from build123d import *

# Parameters (mm, degrees)
SKETCH_1_R             = 19.1
EXTRUDE_1_DEPTH        = 40
SKETCH_2_R             = 5
EXTRUDE_2_DEPTH        = 17
CUT_EXTRUDE_START      = -15
CUT_EXTRUDE_1_DEPTH    = 15
HOLE_WIZARD_M3_1_D     = 2.5
HOLE_WIZARD_M3_1_DEPTH = 8.5
HOLE_WIZARD_M3_1_TIP   = 0.721687836


with BuildPart() as part:
    # 草图1 → 凸台-拉伸1 (new body)
    with BuildSketch(Plane(origin=(0, 0, 0), x_dir=(1, 0, 0), z_dir=(0, 1, 0))):
        with Locations(Location((0, 0, 0), (0, 0, 270))):
            Circle(SKETCH_1_R)
    extrude(amount=EXTRUDE_1_DEPTH)

    # 草图2 → 凸台-拉伸2 (add)
    with BuildSketch(Plane(origin=(0, 40, 0), x_dir=(1, 0, 0), z_dir=(0, 1, 0))):
        with Locations(Location((0, 0, 0), (0, 0, 270))):
            Circle(SKETCH_2_R)
    extrude(amount=EXTRUDE_2_DEPTH)

    # 草图3 → 切除-拉伸1 (cut)
    with BuildSketch(Plane(origin=(0, 57, 0), x_dir=(1, 0, 0), z_dir=(0, 1, 0)).offset(CUT_EXTRUDE_START)):
        with BuildLine():
            Line((-3, 4), (3, 4))
            ThreePointArc((3, 4), (0, 5), (-3, 4))
        make_face()
    extrude(amount=CUT_EXTRUDE_1_DEPTH, mode=Mode.SUBTRACT)

    # M3 螺纹孔1
    with Locations(Plane(origin=(0, 40, -15), x_dir=(0, 0, 1), z_dir=(0, 1, 0))):
        with Locations((0, 0), (15, -15), (15, 15), (30, 0)):
            Hole(HOLE_WIZARD_M3_1_D / 2, depth=HOLE_WIZARD_M3_1_DEPTH)
            with Locations((0, 0, -(HOLE_WIZARD_M3_1_DEPTH + HOLE_WIZARD_M3_1_TIP / 2))):  # 120° drill point
                Cone(0, HOLE_WIZARD_M3_1_D / 2, HOLE_WIZARD_M3_1_TIP, mode=Mode.SUBTRACT)


solid = part.part
Design review of the part built by this model. Coordinates are the model's own, in mm. A direction names the side the tool comes from. Give positions to 0.01 mm unless a question says otherwise; leave off trailing zeros. Loops run counter-clockwise (first coordinate to the right, second up) from the corner with the lowest first, then second, coordinate; pieces in that order, holes last. Notation, with made-up numbers: M -15.75,84.5 L -2.75,84.5 A14 ccw -2.75,93.5 Z; hole C 31.25,66.5 d8. An arc over 180 degrees is marked long. One line per question, with ' | ' between items. Start each with the question number.
1. Add section D-D (y = 4.5). Write out the cut boundary in (x, z), plus the area to 3 significant figures.
2. For faces 4 (the face through (0, 0, 0)), 5 (the face through (0.05, 35.69, -13.75)), list the 3-axis set-ups (+Z, -Z, +X, -X, +Y, -Y) from which the entire face can be reached by the end or side of a thin tool; tool diameter is ignored.
3. Add section C-C (z = 9.5). Write out the cut boundary in (x, y).
4. Add section A-A (x = -4). Write out the cut boundary in (y, z).
5. Add section B-B (y = 46). Write out the cut boundary in (x, z).
6. The part is to be moulded in two halves that separate along X. For faces 1 (the face through (0, 49, -4)), 2 (the face through (5.737, 19.72, 18.218)), 3 (the face through (-0.083, 30.904, -14.799)), say which applies: released by +X, released by -X, zero draft, split by the parting line, or undercut.
7. Insertion check: P1, Ø3, axis at x = 0.5, y = 48.5, coming from the -Z side; P2, Ø4, axis at x = -7.5, y = 27.5, coming from the +Z side; P3, Ø3, axis at x = -15, z = 0, coming from the +Y side. Each pin has a flat end and moves straight along its axis. Give the tip position at first contact, or say it passes through.
8. To check wall thickness, follow L1, parallel to X at y = 34, z = 0; L2, parallel to Y at x = -2.5, z = 7.5; L3, parallel to Z at x = 15, y = 38.25. State the ranges of each line that lie inside material, in increasing order.
Worked out:
1) outline: C 0,0 d38.2 | area: 1,150 mm²
2) face 4: +Z, -Z, +X, -X, -Y | face 5: +Y
3) outline: M -16.57,0 L 16.57,0 L 16.57,40 L -16.57,40 Z
4) outline: M 0,-18.68 L 40,-18.68 L 40,-3 L 57,-3 L 57,3 L 40,3 L 40,18.68 L 0,18.68 Z
5) outline: M -3,-4 L 3,-4 A5 ccw long Z
6) face 1: zero draft | face 2: split by the parting line | face 3: undercut
7) P1: stops at z = -4 | P2: stops at z = 18.29 | P3: stops at y = 40
8) L1: x = -19.1 to -16.25, -13.75 to 13.75, 16.25 to 19.1 | L2: y = 0 to 40 | L3: z = -11.82 to -1.25, 1.25 to 11.82
